from build123d import *

# Parameters (mm, degrees)
F0_R     = 7.62
F1_DEPTH = 1.016
F2_R     = 1.016
F3_DEPTH = 2.286
F4_R     = 1.778
F5_DEPTH = 16.51


with BuildPart() as f1:
    # F0 (on Top) → F1 (new body)
    with BuildSketch(Plane.XY):
        Circle(F0_R)
    extrude(amount=F1_DEPTH)

    # F2 (on face) → F3 (join)
    with BuildSketch(Plane.XY.offset(1.016)):
        with Locations((-5.806038, 0)):
            Circle(F2_R)
    extrude(amount=F3_DEPTH)

    # F4 (on face) → F5 (join)
    with BuildSketch(Plane(origin=(0, 0, 0), x_dir=(1, 0, 0), z_dir=(0, 0, -1))):
        Circle(F4_R)
    extrude(amount=F5_DEPTH)


solid = f1.part
Geometry: final body of the model. Coordinates: model frame, mm. A direction names the side the tool comes from. Coordinates: 2 decimals unless noted, no trailing zeros. Order: outer loops, then holes, each group sorted by start corner. A loop starts at its lowest first (then second) coordinate and runs counter-clockwise, first axis right, second up. Notation, with made-up numbers: M 87,45.25 L 137,45.25 A17 cw 137,60.25 Z; hole C -3,-24.75 d8. An arc over 180 degrees is marked long. One line per question, with ' | ' between items. Start each with the question number.
Item 1: Set-up query: faces 1 (the cylindrical face through (-0.385, 1.736, -8.139)), 2 (the cylindrical face through (-1.65, -7.44, 0.5)), 3 (the cylindrical face through (-6.82, 0.04, 2.14)). Return all of +Z, -Z, +X, -X, +Y, -Y with unobstructed straight access to the full face (end or side cutting, diameter ignored); none if empty.
Item 2: Cut plane D-D, the plane x = 4.5. Return the cut outline in (y, z).
Item 3: Ray query, probe 1 along Z at (x, y) = (-2.5, -4.75); probe 2 along Z at (x, y) = (-1.5, 0.5); probe 3 along Y at (x, z) = (-0.5, -9.75). Return the intervals inside material, ascending. Write a range as [from, to].
Item 4: Cut plane C-C, the plane z = -2.25. Return the cut outline in (x, y), then the cut area to 3 significant figures.
Item 5: Cut plane B-B, the plane x = -0.5. Return the cut outline in (y, z), then the cut area to 3 significant figures.
Item 6: Cut plane A-A, the plane y = 0. Return the cut outline in (x, z), then the cut area to 3 significant figures.
Item 7: Pin query (flat end, axial travel): pin 1 Ø4 at (y, z) = (5, -5) entering from -X; pin 2 Ø8 at (y, z) = (3, -14) entering from -X; pin 3 Ø8 at (x, z) = (2, -5.5) entering from +Y; pin 4 Ø1 at (x, y) = (4, -2) entering from -Z. Return the tip coordinate at first contact, or that it passes through.
A:
1) face 1: -Z | face 2: +Z, -Z | face 3: +Z
2) outline: M -6.15,0 L 6.15,0 L 6.15,1.02 L -6.15,1.02 Z
3) probe 1: z = [0, 1.02] | probe 2: z = [-16.51, 1.02] | probe 3: y = [-1.71, 1.71]
4) outline: C 0,0 d3.56 | area: 9.93 mm2
5) outline: M -7.6,0 L -1.71,0 L -1.71,-16.51 L 1.71,-16.51 L 1.71,0 L 7.6,0 L 7.6,1.02 L -7.6,1.02 Z | area: 71.8 mm2
6) outline: M -7.62,0 L -1.78,0 L -1.78,-16.51 L 1.78,-16.51 L 1.78,0 L 7.62,0 L 7.62,1.02 L -4.79,1.02 L -4.79,3.3 L -6.82,3.3 L -6.82,1.02 L -7.62,1.02 Z | area: 78.8 mm2
7) pin 1: passes through | pin 2: stops at x = -1.78 | pin 3: stops at y = 1.78 | pin 4: stops at z = 0
